Part model, mm, in its own coordinate system. Face numbers are marked on the shaded views. A direction names the side the tool comes from. Give positions to 0.01 mm unless a question says otherwise; leave off trailing zeros. Loops run counter-clockwise (first coordinate to the right, second up) from the corner with the lowest first, then second, coordinate; pieces in that order, holes last. Notation, with made-up numbers: M 56.5,-34 L 94.5,-34 A22 cw 94.5,-25 Z; hole C 77,5 d2. An arc over 180 degrees is marked long. Answer in a Markdown table with one row per item.
from build123d import *

# Parameters (mm, degrees)
SKETCH3_R           = 23.00375504
CUT_EXTRUDE3_DEPTH  = 14.574115143
SKETCH4_R           = 12.15
SKETCH4_R_2         = 2.9
SKETCH4_R_3         = 4.15
SKETCH4_R_4         = 2.1
BOSS_EXTRUDE1_DEPTH = 5
FILLET1_R           = 4


with BuildPart() as part:
    # Sketch1 → Revolve1 (revolve)
    with BuildSketch(Plane.XY, mode=Mode.PRIVATE) as revolve1_sk:
        with BuildLine():
            Line((-50.3, 10), (-50.3, -0.3))
            Line((-50.3, -0.3), (-47.7, -0.3))
            Line((-47.7, -0.3), (-47.7, 10))
            Line((-47.7, 10), (-44.7, 10))
            Line((-44.7, 10), (-44.7, 3))
            ThreePointArc((-44.7, 3), (-41.771067812, -4.071067812), (-34.7, -7))
            Line((-34.7, -7), (-17.15, -7))
            ThreePointArc((-17.15, -7), (-10.078932188, -4.071067812), (-7.15, 3))
            Line((-7.15, 3), (-7.15, 7.574115143))
            Line((-7.15, 7.574115143), (-4.15, 7.574115143))
            Line((-4.15, 7.574115143), (-4.15, -10))
            Line((-4.15, -10), (-48, -10))
            Line((-48, -10), (-53, -5))
            Line((-53, -5), (-53, 10))
            Line((-53, 10), (-50.3, 10))
        make_face()
    revolve(revolve1_sk.sketch.rotate(Axis((0, 0, 0), (0, 1, 0)), 270), axis=Axis((0, 0, 0), (0, 1, 0)))

    # Sketch3 → Cut-Extrude3 (cut)
    with BuildSketch(Plane(origin=(0, 7.574115143, 0), x_dir=(1, 0, 0), z_dir=(0, 1, 0))):
        Circle(SKETCH3_R)
    extrude(amount=-CUT_EXTRUDE3_DEPTH, mode=Mode.SUBTRACT)

    # Sketch4 → Boss-Extrude1 (add)
    # profile 1 of 4: a face of its own
    with BuildSketch(Plane(origin=(0, -7, 0), x_dir=(1, 0, 0), z_dir=(0, 1, 0))):
        with Locations(Location((0, 0, 0), (0, 0, 90))):
            Circle(SKETCH4_R)
        with Locations(Location((7.377762048, -3.462820695, 0), (0, 0, 270))):
            Circle(SKETCH4_R_2, mode=Mode.SUBTRACT)
        with Locations(Location((-0.689990334, 8.120739704, 0), (0, 0, 270))):
            Circle(SKETCH4_R_2, mode=Mode.SUBTRACT)
        with Locations(Location((-6.687771714, -4.657919009, 0), (0, 0, 270))):
            Circle(SKETCH4_R_2, mode=Mode.SUBTRACT)
        with Locations(Location((0, 0, 0), (0, 0, 90))):
            Circle(SKETCH4_R_3, mode=Mode.SUBTRACT)
    # profile 2 of 4: a face of its own
    with BuildSketch(Plane(origin=(0, -7, 0), x_dir=(1, 0, 0), z_dir=(0, 1, 0))):
        with Locations(Location((-6.687771714, -4.657919009, 0), (0, 0, 90))):
            Circle(SKETCH4_R_4)
    # profile 3 of 4: a face of its own
    with BuildSketch(Plane(origin=(0, -7, 0), x_dir=(1, 0, 0), z_dir=(0, 1, 0))):
        with Locations(Location((7.377762048, -3.462820695, 0), (0, 0, 90))):
            Circle(SKETCH4_R_4)
    # profile 4 of 4: a face of its own
    with BuildSketch(Plane(origin=(0, -7, 0), x_dir=(1, 0, 0), z_dir=(0, 1, 0))):
        with Locations(Location((-0.689990334, 8.120739704, 0), (0, 0, 90))):
            Circle(SKETCH4_R_4)
    extrude(amount=BOSS_EXTRUDE1_DEPTH)

    # Fillet1
    fillet1_edges = [part.edges().sort_by_distance(p)[0] for p in [
        (0, -7, 12.15),
    ]]
    fillet(fillet1_edges, radius=FILLET1_R)


solid = part.part
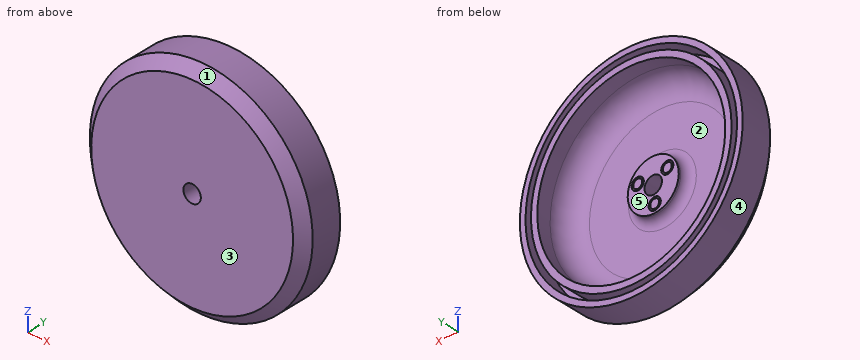
(1) Pull direction Z, two halves, no side cores. Call the marked faces 1, 2 and 3: +Z half, -Z half, draft (parallel to the pull), parting line (faces both ways), or undercut.
Recorded:
| item | result |
|---|---|
| face 1 | parting line |
| face 2 | undercut |
| face 3 | draft |
(2) Drill centre lines: line 1 along X through (y, z) = (6, 0); line 2 along Z through (x, y) = (11.5, 7); line 3 along X through (y, z) = (6, -14.5). Where is each one in solid material? Low to high.
Recorded:
| item | result |
|---|---|
| line 1 | x = -53 to -50.3, -47.7 to -44.7, 44.7 to 47.7, 50.3 to 53 |
| line 2 | z = -51.74 to -48.97, -46.29 to -43.2, 43.2 to 46.29, 48.97 to 51.74 |
| line 3 | x = -50.98 to -48.16, -45.44 to -42.28, 42.28 to 45.44, 48.16 to 50.98 |
(3) Pin check, flat tips, straight feed: pin 1 Ø8 at (y, z) = (7, 13) entering from -X; pin 2 Ø12 at (y, z) = (2, 5) entering from +X; pin 3 Ø12 at (y, z) = (7.5, 18.5) entering from -X. Stop position of each tip, or through.
Recorded:
| item | result |
|---|---|
| pin 1 | stops at x = -52.23 |
| pin 2 | stops at x = 53 |
| pin 3 | stops at x = -51.5 |
(4) Saw through at A-A (y = 6.75). Write the cut outline in (x, z).
Recorded:
| item | result |
|---|---|
| outline | C 0,0 d106; C 0,0 d95.4; hole C 0,0 d100.6; hole C 0,0 d89.4 |
(5) Which spindle directions (+Z, -Z, +X, -X, +Y, -Y) get a long thin tool onto all of the face, cutting with end or side? Do the marked faces 4 and 5. Say none if no direction does.
Recorded:
| item | result |
|---|---|
| face 4 | +Y, -Y |
| face 5 | +Y |
